```python
from build123d import *

# Parameters (mm, degrees)
SKETCH_1_W      = 100
SKETCH_1_H      = 180
EXTRUDE_1_DEPTH = 20
SKETCH_2_W      = 100
SKETCH_2_H      = 110.772585851
EXTRUDE_2_DEPTH = 15
FILLET_1_R      = 10
FILLET_2_R      = 10


with BuildPart() as part:
    # 草图1 → 凸台-拉伸1 (new body)
    with BuildSketch(Plane.XY):
        Rectangle(SKETCH_1_W, SKETCH_1_H)
    extrude(amount=EXTRUDE_1_DEPTH)

    # 草图2 → 凸台-拉伸2 (add)
    with BuildSketch(Plane.XY.offset(20)):
        with Locations((0, -34.613707074)):
            Rectangle(SKETCH_2_W, SKETCH_2_H)
    extrude(amount=EXTRUDE_2_DEPTH)

    # 圆角1
    fillet_1_edges = [part.edges().sort_by_distance(p)[0] for p in [
        (0, 20.772585851, 35),
    ]]
    fillet(fillet_1_edges, radius=FILLET_1_R)

    # 圆角2
    fillet_2_edges = [part.edges().sort_by_distance(p)[0] for p in [
        (0, 20.772585851, 20),
    ]]
    fillet(fillet_2_edges, radius=FILLET_2_R)


solid = part.part
```
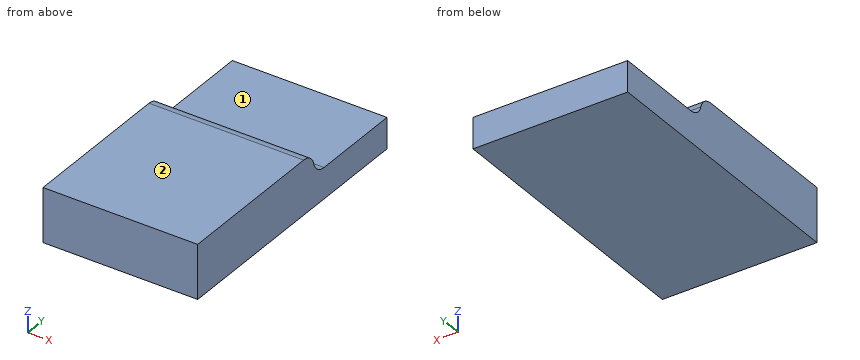
Here's how the part is built. I have some questions about the finished solid (model axes, mm). Face numbers are marked on the shaded views. A direction names the side the tool comes from. Give positions to 0.01 mm unless a question says otherwise; leave off trailing zeros. Write each loop counter-clockwise with the first axis right and the second up, starting at its lowest first coordinate (ties: lowest second). Pieces come first, ordered by that corner, then holes. Notation, with made-up numbers: (31.5, -18) -> (66.5, -18) arc R10 cw to (66.5, -4) -> close; hole circle Ø6 at (29, 41). An arc over 180 degrees is marked (long way). Write each question's results on one line, items separated by ' | '.
Item 1: Suppose I cut it at A-A on y = 36.5. Write out the boundary of the cut face in (x, z), plus the area to 3 significant figures.
Output:
outline: (-50, 0) -> (50, 0) -> (50, 20) -> (-50, 20) -> close | area: 2,000 mm^2
Item 2: For pin 1 Ø4 at (x, y) = (11, 28) entering from +Z; pin 2 Ø4 at (x, y) = (37.5, 55.5) entering from +Z; pin 3 Ø6 at (x, y) = (29.5, 70.5) entering from -Z, each with a flat end and sliding along its axis, tell me the tip position at first contact or that it passes through.
Output:
pin 1: stops at z = 20.9 | pin 2: stops at z = 20 | pin 3: stops at z = 0
Item 3: If I drill on L1, parallel to Z at x = 16, y = 76; L2, parallel to Y at x = -25.5, z = 23; L3, parallel to Y at x = 7, z = 33.5, over which ranges is the centre line in solid material (lowest first)?
Output:
L1: z = 0 to 20 | L2: y = -90 to 23 | L3: y = -90 to 16.04
Item 4: Suppose I cut it at B-B on z = 29.5. Write out the boundary of the cut face in (x, y), plus the area to 3 significant figures.
Output:
outline: (-50, -90) -> (50, -90) -> (50, 19.7) -> (-50, 19.7) -> close | area: 11,000 mm^2
Item 5: On a 3-axis mill with a long thin cutter (end or side, diameter ignored), from which of +Z, -Z, +X, -X, +Y, -Y can I reach the whole of each face in a straight line? I mean the marked faces 1 and 2. Say none if no direction works.
Output:
face 1: +Z, +X, -X, +Y | face 2: +Z, +X, -X, +Y, -Y
